Print and shaded views of the part. All mm, measured from the part's lowest x, y and z. Coordinates: 2 decimals unless noted, no trailing zeros. Loops run counter-clockwise (first coordinate to the right, second up) from the corner with the lowest first, then second, coordinate; pieces in that order, holes last.
1) Saw through at C-C, the plane x = 13. Write the cut outline in (y, z), and give its area (3 significant figures).
2) Saw through at B-B, the plane z = 2.35. Write the cut outline in (x, y), and give its area (3 significant figures).
3) Saw through at A-A, the plane x = 135. Write the cut outline in (y, z).
4) Saw through at D-D, the plane y = 40. Write the cut outline in (x, z).
5) Pin check, flat tip, straight feed: pin 1 Ø1.5 at (y, z) = (44.5, 2.5) entering from -X. Stop position of the tip, or through.
6) Wall check: line 1 along Y through (x, z) = (118, 4); line 2 along Y through (x, z) = (40, 4.7); line 3 along X through (y, z) = (114, 2.95). Give the ranges that are in metal, low to high.
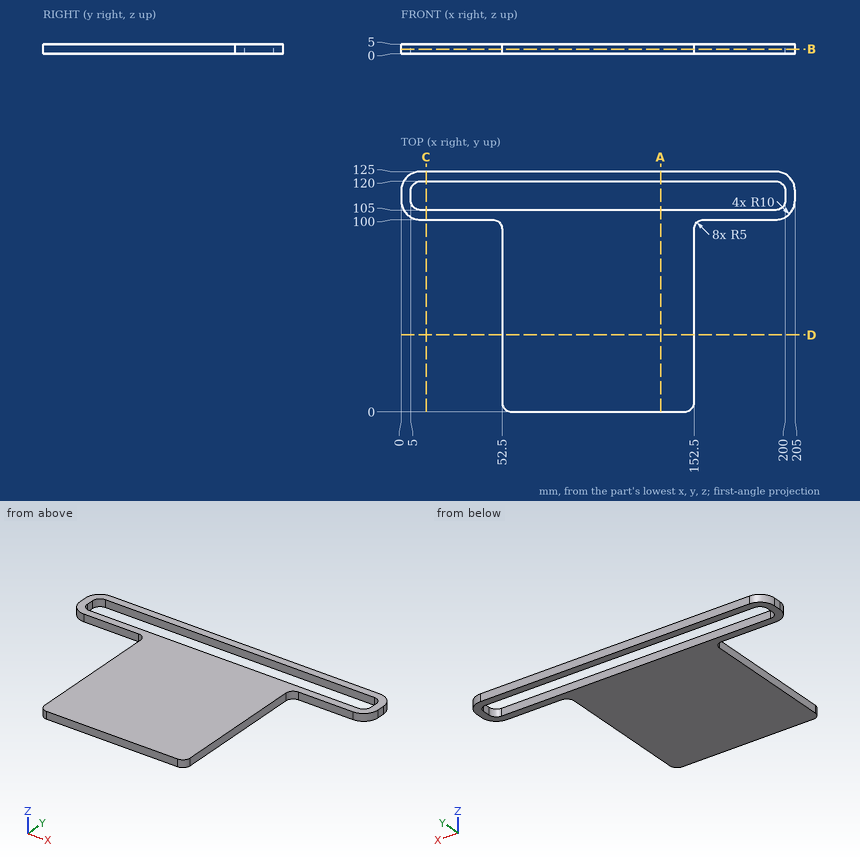
Data:
1. outline: (100, 0) - (105, 0) - (105, 5) - (100, 5) - close; (120, 0) - (125, 0) - (125, 5) - (120, 5) - close
1. area: 50.0 mm2
2. outline: (0, 110) arc R10 ccw to (10, 100) - (47.5, 100) arc R5 cw to (52.5, 95) - (52.5, 5) arc R5 ccw to (57.5, 0) - (147.5, 0) arc R5 ccw to (152.5, 5) - (152.5, 95) arc R5 cw to (157.5, 100) - (195, 100) arc R10 ccw to (205, 110) - (205, 115) arc R10 ccw to (195, 125) - (10, 125) arc R10 ccw to (0, 115) - close; hole (5, 110) arc R5 ccw to (10, 105) - (195, 105) arc R5 ccw to (200, 110) - (200, 115) arc R5 ccw to (195, 120) - (10, 120) arc R5 ccw to (5, 115) - close
2. area: 12,100 mm2
3. outline: (0, 0) - (105, 0) - (105, 5) - (0, 5) - close; (120, 0) - (125, 0) - (125, 5) - (120, 5) - close
4. outline: (52.5, 0) - (152.5, 0) - (152.5, 5) - (52.5, 5) - close
5. pin 1: stops at x = 52.5
6. line 1: y = 0 to 105, 120 to 125
6. line 2: y = 100 to 105, 120 to 125
6. line 3: x = 0 to 5, 200 to 205
